from build123d import *
from build123d.topology import SkipClean

# Parameters (mm, degrees)
IZIM3_R                     = 105
IZIM3_R_2                   = 15
Y_KSEKLIK_EKSTR_ZYON1_DEPTH = 50
IZIM4_R                     = 30
KES_EKSTR_ZYON1_DEPTH       = 10
IZIM5_R                     = 145
IZIM5_R_2                   = 105
EKSTR_ZYON_NCE1_DEPTH       = 100
IZIM95_R                    = 145
IZIM95_R_2                  = 105
RADYUS1_R                   = 10
RADYUS2_R                   = 10


with BuildPart() as part:
    # izim3 → Y_kseklik-Ekstr_zyon1 (new body)
    with BuildSketch(Plane.XY):
        with BuildLine():
            Line((-160, -180), (160, -180))
            ThreePointArc((160, -180), (174.142135624, -174.142135624), (180, -160))
            Line((180, -160), (180, 160))
            ThreePointArc((180, 160), (174.142135624, 174.142135624), (160, 180))
            Line((160, 180), (-160, 180))
            ThreePointArc((-160, 180), (-174.142135624, 174.142135624), (-180, 160))
            Line((-180, 160), (-180, -160))
            ThreePointArc((-180, -160), (-174.142135624, -174.142135624), (-160, -180))
        make_face()
        Circle(IZIM3_R, mode=Mode.SUBTRACT)
        with Locations((-130, 130)):
            Circle(IZIM3_R_2, mode=Mode.SUBTRACT)
        with Locations(Location((130, 130, 0), (0, 0, 180))):
            Circle(IZIM3_R_2, mode=Mode.SUBTRACT)
        with Locations(Location((-130, -130, 0), (0, 0, 180))):
            Circle(IZIM3_R_2, mode=Mode.SUBTRACT)
        with Locations((130, -130)):
            Circle(IZIM3_R_2, mode=Mode.SUBTRACT)
    y_kseklik_ekstr_zyon1 = extrude(amount=-Y_KSEKLIK_EKSTR_ZYON1_DEPTH)

    # izim4 → Kes-Ekstr_zyon1 (cut)
    with BuildSketch(Plane.XY):
        with Locations((-130, 130)):
            Circle(IZIM4_R)
        with Locations((130, 130)):
            Circle(IZIM4_R)
        with Locations((130, -130)):
            Circle(IZIM4_R)
        with Locations((-130, -130)):
            Circle(IZIM4_R)
    kes_ekstr_zyon1 = extrude(amount=-KES_EKSTR_ZYON1_DEPTH, mode=Mode.SUBTRACT)

    # izim5 → Ekstr_zyon-_nce1 (add)
    with SkipClean():  # the faces are left unmerged after this step: merging them gives an invalid solid
        with BuildSketch(Plane(origin=(0, 0, -50), x_dir=(-1, 0, 0), z_dir=(0, 0, -1))):
            Circle(IZIM5_R)
            Circle(IZIM5_R_2, mode=Mode.SUBTRACT)
        ekstr_zyon_nce1 = extrude(amount=EKSTR_ZYON_NCE1_DEPTH)
    add(part.part.scale(1), mode=Mode.REPLACE)  # the faces are merged on a copy

    # S_p_r1: sweep along a path in izim6
    with BuildLine(Plane(origin=(0, 0, 0), x_dir=(0, 0, -1), z_dir=(1, 0, 0))) as s_p_r1_path:
        ThreePointArc((150, 0), (333.847761128, 76.152234911), (410, 259.999994399))
    # izim95 → S_p_r1 (sweep)
    with BuildSketch(Plane(origin=(0, 0, -150), x_dir=(-1, 0, 0), z_dir=(0, 0, -1))):
        Circle(IZIM95_R)
        Circle(IZIM95_R_2, mode=Mode.SUBTRACT)
    sweep(path=s_p_r1_path.line)

    # Aynalama1: Ekstr_zyon-_nce1 across plane
    add(ekstr_zyon_nce1.mirror(Plane(origin=(0, 204.999997199, -205.000001616), x_dir=(0, 0.7071067888032234, 0.7071067735698715), z_dir=(0, 0.7071067735698718, -0.7071067888032233))))

    # Aynalama2: Y_kseklik-Ekstr_zyon1, Kes-Ekstr_zyon1 across plane
    add(y_kseklik_ekstr_zyon1.mirror(Plane(origin=(0, 204.999997199, -205.000001616), x_dir=(0, 0.7071067888032234, 0.7071067735698715), z_dir=(0, 0.7071067735698718, -0.7071067888032233))))
    add(kes_ekstr_zyon1.mirror(Plane(origin=(0, 204.999997199, -205.000001616), x_dir=(0, 0.7071067888032234, 0.7071067735698715), z_dir=(0, 0.7071067735698718, -0.7071067888032233))), mode=Mode.SUBTRACT)

    # Radyus1
    radyus1_edges = [part.edges().sort_by_distance(p)[0] for p in [
        (-174.142135624, 359.999990647, -584.142137778),
        (0, 359.999990521, -590.000002154),
        (174.142135624, 359.999990647, -584.142137778),
        (180, 359.999994399, -410.000002154),
        (174.142135624, 359.99999815, -235.857866531),
        (0, 359.999998277, -230.000002154),
        (-174.142135624, 359.99999815, -235.857866531),
        (-180, 359.999994399, -410.000002154),
    ]]
    fillet(radyus1_edges, radius=RADYUS1_R)

    # Radyus2
    radyus2_edges = [part.edges().sort_by_distance(p)[0] for p in [
        (174.142135624, -174.142135624, -50),
        (180, 0, -50),
        (174.142135624, 174.142135624, -50),
        (0, 180, -50),
        (-174.142135624, 174.142135624, -50),
        (-180, 0, -50),
        (-174.142135624, -174.142135624, -50),
        (0, -180, -50),
    ]]
    fillet(radyus2_edges, radius=RADYUS2_R)


solid = part.part
Design review of the part built by this model. Coordinates are the model's own, in mm. A direction names the side the tool comes from. Coordinates: 2 decimals unless noted, no trailing zeros. Order: outer loops, then holes, each group sorted by start corner. A loop starts at its lowest first (then second) coordinate and runs counter-clockwise, first axis right, second up. Notation, with made-up numbers: (45.25, 48) -> (74.25, 48) arc R33 cw to (74.25, 84) -> close; hole circle Ø2 at (76, 10). An arc over 180 degrees is marked (long way). Use one line per item in the form item = value. Start each with the question number.
(1) For faces 4 (the flat face through (136, 144, -10)), 5 (the flat face through (136, 400, -526)), 6 (the cylindrical face through (-138.304, 43.554, -99.3)), list the 3-axis set-ups (+Z, -Z, +X, -X, +Y, -Y) from which the entire face can be reached by the end or side of a thin tool; tool diameter is ignored.
(2) Add section D-D on x = -45.5. State the section outline as (y, z) points, plus the area to 3 significant figures.
(3) Add section A-A on x = 0. State the section outline as (y, z) points, plus the area to 3 significant figures.
(4) The part is to be moulded in two halves that separate along X. For faces 1 (the flat face through (-2, 390, -590)), 2 (the cylindrical face through (126.095, 405.07, -510.255)), 3 (the flat face through (180, 390, -412)), say which applies: +X half, -X half, draft (parallel to the pull), parting line (faces both ways), or undercut.
(5) Insertion check: pin 1 (12 mm diameter, centred on x = -32.5, z = -20, fed in from +Y); pin 2 (20 mm diameter, centred on x = -21.5, y = 390, fed in from +Z); pin 3 (4 mm diameter, centred on x = -36.5, z = -205, fed in from +Y) (3 decimals). Each pin has a flat end and moves straight along its axis. Give the tip position at first contact, or say it passes through.
(6) For probe 1 along Z at (x, y) = (130, 407); probe 2 along Y at (x, z) = (130, -2.25); probe 3 along Y at (x, z) = (130, -30), list the stretches that pass through material, from the lowest coordinate up.
(7) Add section C-C on y = 130. Give the number of separate pieces and of enclosed holes in the cut face, plus the area to 3 significant figures.
(8) Add section B-B on z = -92. State the section outline as (x, y) points, plus the area to 3 significant figures.
Answer block:
q1.face_4 = +Z
q1.face_5 = +Y
q1.face_6 = none
q2.outline = (-180, -40) arc R10 ccw to (-170, -50) -> (-137.68, -50) -> (-137.68, -150) arc R397.68 ccw to (260, -547.68) -> (360, -547.68) -> (360, -580) arc R10 ccw to (370, -590) -> (410, -590) -> (410, -504.63) -> (260, -504.63) arc R354.63 cw to (-94.63, -150) -> (-94.63, 0) -> (-180, 0) -> close; (94.63, -150) arc R165.37 ccw to (260, -315.37) -> (410, -315.37) -> (410, -230) -> (370, -230) arc R10 ccw to (360, -240) -> (360, -272.32) -> (260, -272.32) arc R122.32 cw to (137.68, -150) -> (137.68, -50) -> (170, -50) arc R10 ccw to (180, -40) -> (180, 0) -> (94.63, 0) -> close
q2.area = 69,400 mm²
q3.outline = (-180, -40) arc R10 ccw to (-170, -50) -> (-145, -50) -> (-145, -150) arc R405 ccw to (260, -555) -> (360, -555) -> (360, -580) arc R10 ccw to (370, -590) -> (410, -590) -> (410, -515) -> (260, -515) arc R365 cw to (-105, -150) -> (-105, 0) -> (-180, 0) -> close; (105, -150) arc R155 ccw to (260, -305) -> (410, -305) -> (410, -230) -> (370, -230) arc R10 ccw to (360, -240) -> (360, -265) -> (260, -265) arc R115 cw to (145, -150) -> (145, -50) -> (170, -50) arc R10 ccw to (180, -40) -> (180, 0) -> (105, 0) -> close
q3.area = 63,600 mm²
q4.face_1 = draft
q4.face_2 = undercut
q4.face_3 = +X half
q5.pin_1 = 180
q5.pin_2 = -230
q5.pin_3 = 154.925
q6.probe_1 = -590 to -570, -510 to -310, -250 to -230
q6.probe_2 = -180 to -160, -100 to 100, 160 to 180
q6.probe_3 = -180 to -145, -115 to 115, 145 to 180
q7.separate_pieces = 3
q7.enclosed_holes = 1
q7.area = 71,500 mm²
q8.outline = circle Ø290 at (0, 0); hole circle Ø210 at (0, 0)
q8.area = 31,400 mm²
